from build123d import *

# Parameters (mm, degrees)
SKETCH_1_W                   = 40
SKETCH_1_H                   = 40
SKETCH_1_R                   = 5.2
SKETCH_1_R_2                 = 1.6
EXTRUDE_1_DEPTH              = 5
HOLE_WIZARD_1_D              = 3
CHAMFER_1_SIZE               = 2
HOLE_WIZARD_M3_2_D           = 3.4
HOLE_WIZARD_M3_2_CSINK_D     = 6.6
HOLE_WIZARD_M3_2_CSINK_ANGLE = 90
SKETCH_7_R                   = 2.5
EXTRUDE_2_DEPTH              = 5
SKETCH_10_W                  = 9
SKETCH_10_H                  = 7
SKETCH_10_R                  = 1.5
EXTRUDE_4_DEPTH              = 4
EXTRUDE_6_DEPTH              = 3
SKETCH_13_W                  = 13.015545452
SKETCH_13_H                  = 100
SKETCH_13_R                  = 2.6
SKETCH_13_R_2                = 1.5
EXTRUDE_7_DEPTH              = 5
HOLE_WIZARD_M3_3_D           = 3.4
HOLE_WIZARD_M3_3_CSINK_D     = 6.6
HOLE_WIZARD_M3_3_CSINK_ANGLE = 90


with BuildPart() as part:
    # 草图1 → 凸台-拉伸1 (new body)
    with BuildSketch(Plane.XY):
        Rectangle(SKETCH_1_W, SKETCH_1_H)
        Circle(SKETCH_1_R, mode=Mode.SUBTRACT)
        with Locations((5.656854249, 5.656854249)):
            Circle(SKETCH_1_R_2, mode=Mode.SUBTRACT)
        with Locations((5.656854249, -5.656854249)):
            Circle(SKETCH_1_R_2, mode=Mode.SUBTRACT)
        with Locations((-5.656854249, -5.656854249)):
            Circle(SKETCH_1_R_2, mode=Mode.SUBTRACT)
        with Locations((-5.656854249, 5.656854249)):
            Circle(SKETCH_1_R_2, mode=Mode.SUBTRACT)
    extrude(amount=EXTRUDE_1_DEPTH)

    # 孔1 (through all)
    with Locations(Plane(origin=(16.25, -4, 5), x_dir=(1, 0, 0), z_dir=(0, 0, 1))):
        with Locations((0, 0), (-32.5, 0)):
            Hole(HOLE_WIZARD_1_D / 2)

    # 倒角1
    chamfer_1_edges = [part.edges().sort_by_distance(p)[0] for p in [
        (20, 20, 2.5),
    ]]
    chamfer(chamfer_1_edges, length=CHAMFER_1_SIZE)

    # M3 十字槽沉头木螺钉的锥形沉头孔2 (through all)
    with Locations(Plane.XY.offset(5)):
        with Locations((-5.656854249, 5.656854249), (5.656854249, 5.656854249), (5.656854249, -5.656854249), (-5.656854249, -5.656854249)):
            CounterSinkHole(HOLE_WIZARD_M3_2_D / 2, HOLE_WIZARD_M3_2_CSINK_D / 2, counter_sink_angle=HOLE_WIZARD_M3_2_CSINK_ANGLE)

    # 草图7 → 凸台-拉伸2 (add)
    with BuildSketch(Plane(origin=(0, 0, 0), x_dir=(-1, 0, 0), z_dir=(0, 0, -1))):
        Polygon((-11.507772726, 20), (-6.507772726, 20), (6.507772726, 20), (11.507772726, 20), (6.507772726, 32), (-6.507772726, 32), align=None)
        with Locations((0, 26)):
            Circle(SKETCH_7_R, mode=Mode.SUBTRACT)
    extrude(amount=-EXTRUDE_2_DEPTH)

    # 草图10 → 凸台-拉伸4 (add)
    with BuildSketch(Plane.XZ.offset(20)):
        with Locations((15.5, -3.5)):
            Rectangle(SKETCH_10_W, SKETCH_10_H)
        with Locations(Location((17, -4, 0), (0, 0, 270))):
            Circle(SKETCH_10_R, mode=Mode.SUBTRACT)
    extrude_4 = extrude(amount=-EXTRUDE_4_DEPTH)

    # 草图12 → 凸台-拉伸6 (add)
    with BuildSketch(Plane.ZY.offset(-11)):
        Polygon((-7, -16), (0, -9), (0, -16), align=None)
    extrude_6 = extrude(amount=-EXTRUDE_6_DEPTH)

    # 镜向2: 凸台-拉伸4, 凸台-拉伸6 across plane
    add(extrude_4.mirror(Plane(origin=(0, 0, 0), x_dir=(0, 0, 1), z_dir=(1, 0, 0))))
    add(extrude_6.mirror(Plane(origin=(0, 0, 0), x_dir=(0, 0, 1), z_dir=(1, 0, 0))))

    # 草图13 → 凸台-拉伸7 (add)
    with BuildSketch(Plane.XY.offset(5)):
        with Locations((0, 82)):
            Rectangle(SKETCH_13_W, SKETCH_13_H)
        with Locations((0, 122)):
            Circle(SKETCH_13_R, mode=Mode.SUBTRACT)
        with Locations((0, 99)):
            Circle(SKETCH_13_R_2, mode=Mode.SUBTRACT)
        with Locations((0, 73)):
            Circle(SKETCH_13_R_2, mode=Mode.SUBTRACT)
    extrude(amount=-EXTRUDE_7_DEPTH)

    # M3 十字槽沉头木螺钉的锥形沉头孔3 (through all)
    with Locations(Plane.XY.offset(5)):
        with Locations((0, 99), (0, 73)):
            CounterSinkHole(HOLE_WIZARD_M3_3_D / 2, HOLE_WIZARD_M3_3_CSINK_D / 2, counter_sink_angle=HOLE_WIZARD_M3_3_CSINK_ANGLE)


solid = part.part
The model under review builds one solid part; all positions refer to its coordinate system, in mm. A direction names the side the tool comes from. Round coordinates to 2 decimals unless told otherwise and drop trailing zeros. Write each loop counter-clockwise with the first axis right and the second up, starting at its lowest first coordinate (ties: lowest second). Pieces come first, ordered by that corner, then holes. Notation, with made-up numbers: (71.5, -11) -> (98.5, -11) arc R14 ccw to (98.5, -7) -> close; hole circle Ø10 at (22.25, 35.5). An arc over 180 degrees is marked (long way). Answer as a JSON object with one key per item and string values.
1. We need section A-A on x = 0. State the section outline as (y, z) points, and give its area (3 significant figures).
Results found:
{"outline": "(-20, 0) -> (-5.2, 0) -> (-5.2, 5) -> (-20, 5) -> close; (5.2, 0) -> (23.5, 0) -> (23.5, 5) -> (5.2, 5) -> close; (28.5, 0) -> (71.3, 0) -> (71.3, 3.4) -> (69.7, 5) -> (28.5, 5) -> close; (74.7, 0) -> (97.3, 0) -> (97.3, 3.4) -> (95.7, 5) -> (76.3, 5) -> (74.7, 3.4) -> close; (100.7, 0) -> (119.4, 0) -> (119.4, 5) -> (102.3, 5) -> (100.7, 3.4) -> close; (124.6, 0) -> (132, 0) -> (132, 5) -> (124.6, 5) -> close", "area": "618 mm^2"}
2. To check wall thickness, follow line 1 along X through (y, z) = (99, 2.2); line 2 along X through (y, z) = (-3, 1.75); line 3 along X through (y, z) = (0, 1.9). State the ranges of each line that lie inside material, in increasing order.
Results found:
{"line 1": "x = -6.51 to -1.7, 1.7 to 6.51", "line 2": "x = -20 to -17.37, -15.13 to -4.25, 4.25 to 15.13, 17.37 to 20", "line 3": "x = -20 to -5.2, 5.2 to 20"}
3. We need section C-C on y = 122. State the section outline as (x, z) points.
Results found:
{"outline": "(-6.51, 0) -> (-2.6, 0) -> (-2.6, 5) -> (-6.51, 5) -> close; (2.6, 0) -> (6.51, 0) -> (6.51, 5) -> (2.6, 5) -> close"}
4. Clearance check with flat-ended pins moving along their axes: pin 1 (3 mm diameter, centred on x = 0, y = 122, fed in from -Z); pin 2 (5 mm diameter, centred on x = -17, z = -4, fed in from +Y); pin 3 (2.5 mm diameter, centred on x = -14, z = 3, fed in from +Y); pin 4 (12 mm diameter, centred on x = 6.5, y = 38, fed in from -Z). State where each tip first meets the part, or that it passes through.
Results found:
{"pin 1": "passes through", "pin 2": "stops at y = -16", "pin 3": "stops at y = 20", "pin 4": "stops at z = 0"}
5. The part is to be moulded in two halves that separate along Z. For faces 1 (the face through (0, 40, 0)), 2 (the face through (18.265, -18.028, -4.806)), 3 (the face through (0, 132, 3)), 4 (the face through (0, 40, 5)), say which applies: pulls with the +Z half, pulls with the -Z half, needs draft (parallel to the pull), parting line crosses it, or undercut.
Results found:
{"face 1": "pulls with the -Z half", "face 2": "undercut", "face 3": "needs draft", "face 4": "pulls with the +Z half"}
6. We need section B-B on y = 0. State the section outline as (x, z) points.
Results found:
{"outline": "(-20, 0) -> (-5.2, 0) -> (-5.2, 5) -> (-20, 5) -> close; (5.2, 0) -> (20, 0) -> (20, 5) -> (5.2, 5) -> close"}
7. We need section D-D on y = 85. State the section outline as (x, z) points.
Results found:
{"outline": "(-6.51, 0) -> (6.51, 0) -> (6.51, 5) -> (-6.51, 5) -> close"}
8. Machinability: for faces 5 (the face through (6.508, 81, 3)), 6 (the face through (-16, 20, 2)), 7 (the face through (4.96, 1.56, 2.47)), 8 (the face through (-11, -16, -3)), 9 (the face through (-17, -16, -2)), which of the approach directions +Z, -Z, +X, -X, +Y, -Y give a long, thin tool a straight path to every point of the face, cutting with its end or side? Answer none if there is none.
Results found:
{"face 5": "+Z, -Z, +X, +Y", "face 6": "+Z, -Z, -X, +Y", "face 7": "+Z, -Z", "face 8": "-Z, +Y, -Y", "face 9": "-Z, -X, +Y"}
